Study the drawing (mm; zero at the part's minimum x, y, z) and answer. A direction names the side the tool comes from. Round coordinates to 2 decimals unless told otherwise and drop trailing zeros. Write each loop counter-clockwise with the first axis right and the second up, starting at its lowest first coordinate (ties: lowest second). Pieces come first, ordered by that corner, then holes. Notation, with made-up numbers: (39.5, -18) -> (50.5, -18) arc R28 ccw to (50.5, 7) -> close; hole circle Ø4 at (70.5, 87). An arc over 180 degrees is marked (long way). One line per question, with ' | ' between items. Start each with the question number.
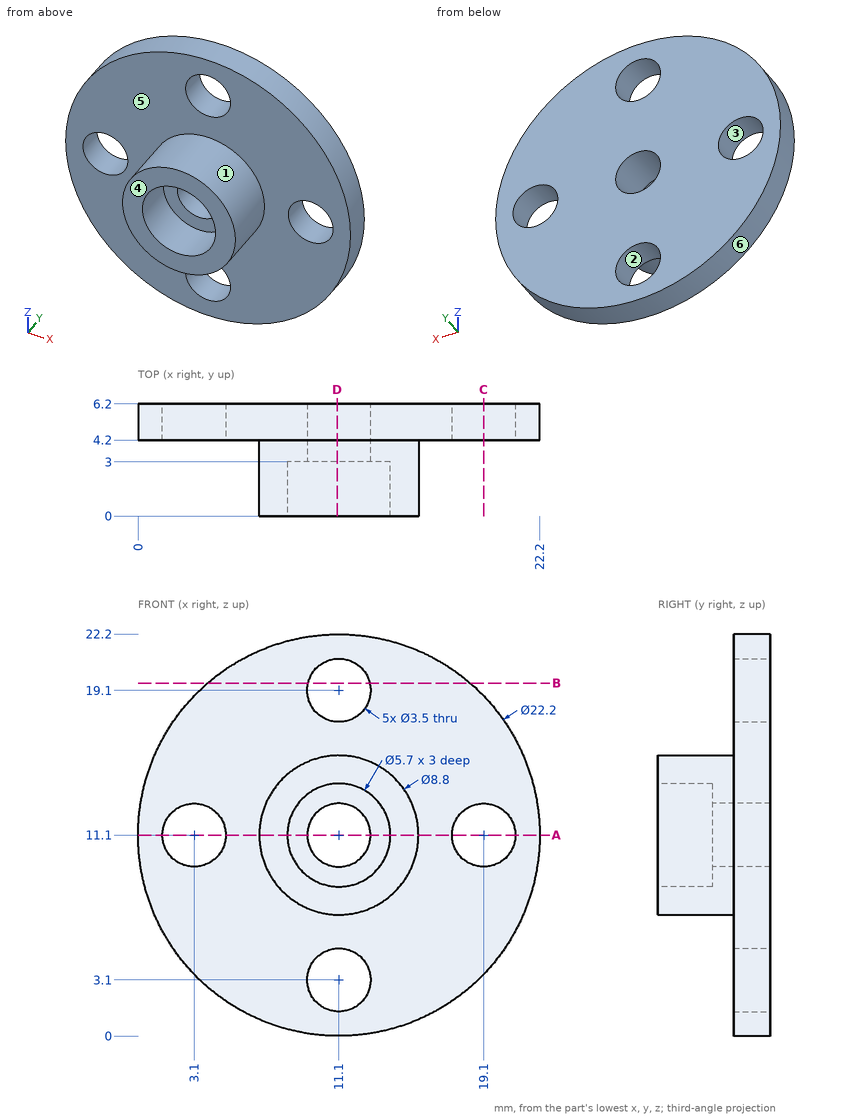
(1) A cutting plane is placed at A-A, the plane z = 11.1. Determine the outline of the cut face in (x, y).
(2) A cutting plane is placed at D-D, the plane x = 11. Determine the outline of the cut face in (y, z).
(3) A cutting plane is placed at C-C, the plane x = 19.1. Determine the outline of the cut face in (y, z), then the cut area to 3 significant figures.
(4) The mould has two halves that part along Z. Classify the marked faces 1, 2, 3 and 4: +Z half, -Z half, draft (parallel to the pull), parting line (faces both ways), or undercut.
(5) Given pin 1 Ø9 at (x, z) = (11.1, 11.1) entering from -Y; pin 2 Ø1 at (x, y) = (7, 5) entering from +Z; pin 3 Ø2 at (x, z) = (11.1, 19.1) entering from -Y; pin 4 Ø5.5 at (x, z) = (19.1, 11.1) entering from -Y, each flat-ended and moving along its own axis, determine where each tip first touches the part or whether it passes through.
(6) A cutting plane is placed at B-B, the plane z = 19.5. Determine the outline of the cut face in (x, y).
(7) Consider L1, parallel to X at y = 5, z = 11; L2, parallel to Z at x = 9.75, y = 5.5. Determine where each line is inside the solid, lowest interval first.
(8) For the marked faces 5 and 6, determine the directions among +Z, -Z, +X, -X, +Y, -Y from which every point of the face is accessible in a straight line to the end or side of a thin tool.
Returned:
1) outline: (0, 4.2) -> (1.35, 4.2) -> (1.35, 6.2) -> (0, 6.2) -> close; (4.85, 4.2) -> (6.7, 4.2) -> (6.7, 0) -> (8.25, 0) -> (8.25, 3) -> (9.35, 3) -> (9.35, 6.2) -> (4.85, 6.2) -> close; (12.85, 3) -> (13.95, 3) -> (13.95, 0) -> (15.5, 0) -> (15.5, 4.2) -> (17.35, 4.2) -> (17.35, 6.2) -> (12.85, 6.2) -> close; (20.85, 4.2) -> (22.2, 4.2) -> (22.2, 6.2) -> (20.85, 6.2) -> close
2) outline: (0, 6.7) -> (4.2, 6.7) -> (4.2, 4.85) -> (6.2, 4.85) -> (6.2, 9.35) -> (3, 9.35) -> (3, 8.25) -> (0, 8.25) -> close; (0, 13.95) -> (3, 13.95) -> (3, 12.85) -> (6.2, 12.85) -> (6.2, 17.35) -> (4.2, 17.35) -> (4.2, 15.5) -> (0, 15.5) -> close; (4.2, 0) -> (6.2, 0) -> (6.2, 1.35) -> (4.2, 1.35) -> close; (4.2, 20.85) -> (6.2, 20.85) -> (6.2, 22.2) -> (4.2, 22.2) -> close
3) outline: (4.2, 3.41) -> (6.2, 3.41) -> (6.2, 9.35) -> (4.2, 9.35) -> close; (4.2, 12.85) -> (6.2, 12.85) -> (6.2, 18.79) -> (4.2, 18.79) -> close | area: 23.8 mm2
4) face 1: parting line | face 2: undercut | face 3: undercut | face 4: draft
5) pin 1: y = 0 | pin 2: z = 21.6 | pin 3: through | pin 4: y = 4.2
6) outline: (3.84, 4.2) -> (9.4, 4.2) -> (9.4, 6.2) -> (3.84, 6.2) -> close; (12.8, 4.2) -> (18.36, 4.2) -> (18.36, 6.2) -> (12.8, 6.2) -> close
7) L1: 0 to 1.35, 4.85 to 9.35, 12.85 to 17.35, 20.85 to 22.2 | L2: 0.08 to 1.99, 4.21 to 9.99, 12.21 to 17.99, 20.21 to 22.12
8) face 5: -Y | face 6: +Y, -Y
